Check sheet for the modelled part. Datum: model origin and axes. Units: mm. Face numbers are marked on the shaded views. A direction names the side the tool comes from. Coordinates: 2 decimals unless noted, no trailing zeros. Loops run counter-clockwise (first coordinate to the right, second up) from the corner with the lowest first, then second, coordinate; pieces in that order, holes last. Notation, with made-up numbers: (65, 79.5) - (118, 79.5) arc R28 cw to (118, 117.5) - close; hole circle Ø10 at (68, 68). An arc over 180 degrees is marked (long way). Write each question's results on one line, items separated by ' | '. Start each with the question number.
1. Gauge pin test, flat end, axial feed: P1, Ø4, axis at x = -6.5, y = -14.5, coming from the +Z side. Record the tip position at first contact, or that the pin passes through.
2. Thickness scan on line 1 (X direction, y = -14.5, z = 0.5); line 2 (X direction, y = 15.5, z = 9.25); line 3 (X direction, y = -4.5, z = 9). Record the ranges inside material, lowest first. Write a range as [from, to].
3. Cross-section at B-B (z = 8.5). Record the cut outline in (x, y).
4. Tool access check on the marked faces 1 and 2. Record the directions out of +Z, -Z, +X, -X, +Y, -Y that give a thin tool (end or side, any length) a straight path to the whole face; none if there is none.
5. Cross-section at C-C (y = 16.5). Record the cut outline in (x, z).
6. Cross-section at A-A (y = 9). Record the cut outline in (x, z), and give its area (3 significant figures).
7. Draft check along Y on the marked faces 3, 4, 5 and 6. Enter one of: released by +Y, released by -Y, zero draft, split by the parting line, or undercut.
8. Cross-section at D-D (x = -28). Record the cut outline in (y, z).
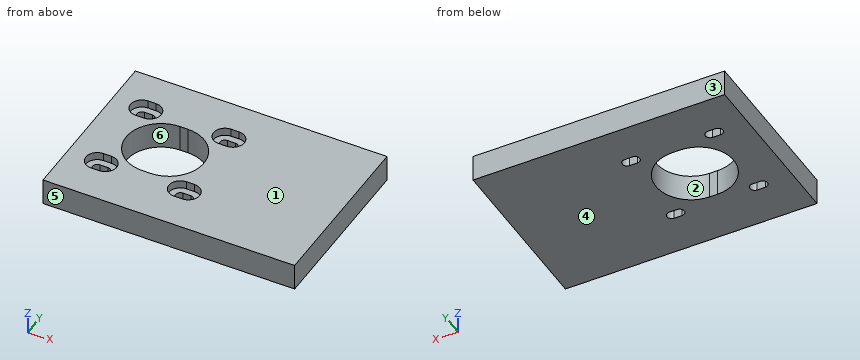
```python
from build123d import *

# Parameters (mm, degrees)
SKETCH1_W           = 93.911938319
SKETCH1_H           = 64.237222829
BOSS_EXTRUDE1_DEPTH = 10
CUT_EXTRUDE1_DEPTH  = 20
CUT_EXTRUDE2_DEPTH  = 3


with BuildPart() as part:
    # Sketch1 → Boss-Extrude1 (new body)
    with BuildSketch(Plane.XY):
        with Locations((-3.99305407, -0.113373268)):
            Rectangle(SKETCH1_W, SKETCH1_H)
    extrude(amount=BOSS_EXTRUDE1_DEPTH)

    # Sketch2 → Cut-Extrude1 (cut)
    with BuildSketch(Plane.XY.offset(10)):
        with BuildLine():
            Line((-39.949023229, 17.755238146), (-36.949023229, 17.755238146))
            ThreePointArc((-36.949023229, 17.755238146), (-35.199023229, 16.005238146), (-36.949023229, 14.255238146))
            Line((-36.949023229, 14.255238146), (-39.949023229, 14.255238146))
            ThreePointArc((-39.949023229, 14.255238146), (-41.699023229, 16.005238146), (-39.949023229, 17.755238146))
        make_face()
        with BuildLine():
            Line((-8.949023229, 17.755238146), (-5.949023229, 17.755238146))
            ThreePointArc((-5.949023229, 17.755238146), (-4.199023229, 16.005238146), (-5.949023229, 14.255238146))
            Line((-5.949023229, 14.255238146), (-8.949023229, 14.255238146))
            ThreePointArc((-8.949023229, 14.255238146), (-10.699023229, 16.005238146), (-8.949023229, 17.755238146))
        make_face()
        with BuildLine():
            Line((-8.949023229, -13.244761854), (-5.949023229, -13.244761854))
            ThreePointArc((-5.949023229, -13.244761854), (-4.199023229, -14.994761854), (-5.949023229, -16.744761854))
            Line((-5.949023229, -16.744761854), (-8.949023229, -16.744761854))
            ThreePointArc((-8.949023229, -16.744761854), (-10.699023229, -14.994761854), (-8.949023229, -13.244761854))
        make_face()
        with BuildLine():
            Line((-39.949023229, -13.244761854), (-36.949023229, -13.244761854))
            ThreePointArc((-36.949023229, -13.244761854), (-35.199023229, -14.994761854), (-36.949023229, -16.744761854))
            Line((-36.949023229, -16.744761854), (-39.949023229, -16.744761854))
            ThreePointArc((-39.949023229, -16.744761854), (-41.699023229, -14.994761854), (-39.949023229, -13.244761854))
        make_face()
        with BuildLine():
            Line((-24.449023229, 13.505238146), (-21.449023229, 13.505238146))
            ThreePointArc((-21.449023229, 13.505238146), (-8.449023229, 0.505238146), (-21.449023229, -12.494761854))
            Line((-21.449023229, -12.494761854), (-24.449023229, -12.494761854))
            ThreePointArc((-24.449023229, -12.494761854), (-37.449023229, 0.505238146), (-24.449023229, 13.505238146))
        make_face()
    extrude(amount=-CUT_EXTRUDE1_DEPTH, mode=Mode.SUBTRACT)

    # Sketch3 → Cut-Extrude2 (cut)
    with BuildSketch(Plane.XY.offset(10)):
        with BuildLine():
            Line((-36.949023229, 20.255238146), (-39.949023229, 20.255238146))
            ThreePointArc((-39.949023229, 20.255238146), (-44.199023229, 16.005238146), (-39.949023229, 11.755238146))
            Line((-39.949023229, 11.755238146), (-36.949023229, 11.755238146))
            ThreePointArc((-36.949023229, 11.755238146), (-32.699023229, 16.005238146), (-36.949023229, 20.255238146))
        make_face()
        with BuildLine():
            Line((-5.949023229, 20.255238146), (-8.949023229, 20.255238146))
            ThreePointArc((-8.949023229, 20.255238146), (-13.199023229, 16.005238146), (-8.949023229, 11.755238146))
            Line((-8.949023229, 11.755238146), (-5.949023229, 11.755238146))
            ThreePointArc((-5.949023229, 11.755238146), (-1.699023229, 16.005238146), (-5.949023229, 20.255238146))
        make_face()
        with BuildLine():
            Line((-5.949023229, -10.744761854), (-8.949023229, -10.744761854))
            ThreePointArc((-8.949023229, -10.744761854), (-13.199023229, -14.994761854), (-8.949023229, -19.244761854))
            Line((-8.949023229, -19.244761854), (-5.949023229, -19.244761854))
            ThreePointArc((-5.949023229, -19.244761854), (-1.699023229, -14.994761854), (-5.949023229, -10.744761854))
        make_face()
        with BuildLine():
            Line((-39.949023229, -19.244761854), (-36.949023229, -19.244761854))
            ThreePointArc((-36.949023229, -19.244761854), (-32.699023229, -14.994761854), (-36.949023229, -10.744761854))
            Line((-36.949023229, -10.744761854), (-39.949023229, -10.744761854))
            ThreePointArc((-39.949023229, -10.744761854), (-44.199023229, -14.994761854), (-39.949023229, -19.244761854))
        make_face()
    extrude(amount=-CUT_EXTRUDE2_DEPTH, mode=Mode.SUBTRACT)


solid = part.part
```
Established:
1) P1: z = 7
2) line 1: [-50.95, -41.63], [-35.27, -10.63], [-4.27, 42.96] | line 2: [-50.95, -44.17], [-32.73, -13.17], [-1.73, 42.96] | line 3: [-50.95, -36.45], [-9.45, 42.96]
3) outline: (-50.95, -32.23) - (42.96, -32.23) - (42.96, 32.01) - (-50.95, 32.01) - close; hole (-39.95, -19.24) - (-36.95, -19.24) arc R4.25 ccw to (-36.95, -10.74) - (-39.95, -10.74) arc R4.25 ccw to start; hole (-39.95, 11.76) - (-36.95, 11.76) arc R4.25 ccw to (-36.95, 20.26) - (-39.95, 20.26) arc R4.25 ccw to start; hole (-24.45, -12.49) - (-21.45, -12.49) arc R13 ccw to (-21.45, 13.51) - (-24.45, 13.51) arc R13 ccw to start; hole (-8.95, -19.24) - (-5.95, -19.24) arc R4.25 ccw to (-5.95, -10.74) - (-8.95, -10.74) arc R4.25 ccw to start; hole (-8.95, 11.76) - (-5.95, 11.76) arc R4.25 ccw to (-5.95, 20.26) - (-8.95, 20.26) arc R4.25 ccw to start
4) face 1: +Z, +X, -X, +Y, -Y | face 2: +Z, -Z
5) outline: (-50.95, 0) - (-41.63, 0) - (-41.63, 7) - (-44.17, 7) - (-44.17, 10) - (-50.95, 10) - close; (-35.27, 0) - (-10.63, 0) - (-10.63, 7) - (-13.17, 7) - (-13.17, 10) - (-32.73, 10) - (-32.73, 7) - (-35.27, 7) - close; (-4.27, 0) - (42.96, 0) - (42.96, 10) - (-1.73, 10) - (-1.73, 7) - (-4.27, 7) - close
6) outline: (-50.95, 0) - (-34.29, 0) - (-34.29, 10) - (-50.95, 10) - close; (-11.61, 0) - (42.96, 0) - (42.96, 10) - (-11.61, 10) - close | area: 712 mm^2
7) face 3: released by +Y | face 4: zero draft | face 5: released by -Y | face 6: undercut
8) outline: (-32.23, 0) - (-12, 0) - (-12, 10) - (-32.23, 10) - close; (13.01, 0) - (32.01, 0) - (32.01, 10) - (13.01, 10) - close
